Here's the drawing with two shaded views (mm, measured from the low corner). I have some questions. Coordinates: 2 decimals unless noted, no trailing zeros. Loops run counter-clockwise (first coordinate to the right, second up) from the corner with the lowest first, then second, coordinate; pieces in that order, holes last. Notation, with made-up numbers: (-36, 53) -> (1, 53) arc R16 cw to (1, 63) -> close; hole circle Ø3 at (89.5, 85.5). An arc over 180 degrees is marked (long way). Answer as a JSON object with one key per item and string values. Group by question number.
1) I want a section at A-A (y = 1.5). Write out the boundary of the cut face in (x, z).
2) I'm going to push a flat-ended pin straight in: pin 1 (1.5 mm diameter, centred on x = 48.5, y = 1.5, fed in from -Z). Where does the tip first touch, or does it pass through?
3) I need wall thicknesses on probe 1 along X at (y, z) = (1.05, 11); probe 2 along Z at (x, y) = (45, 0.45). Which ranges of each line are inside material? Lowest first, please. Write a range as [from, to].
4) I want a section at B-B (x = 84). Write out the boundary of the cut face in (y, z), then the cut area to 3 significant figures.
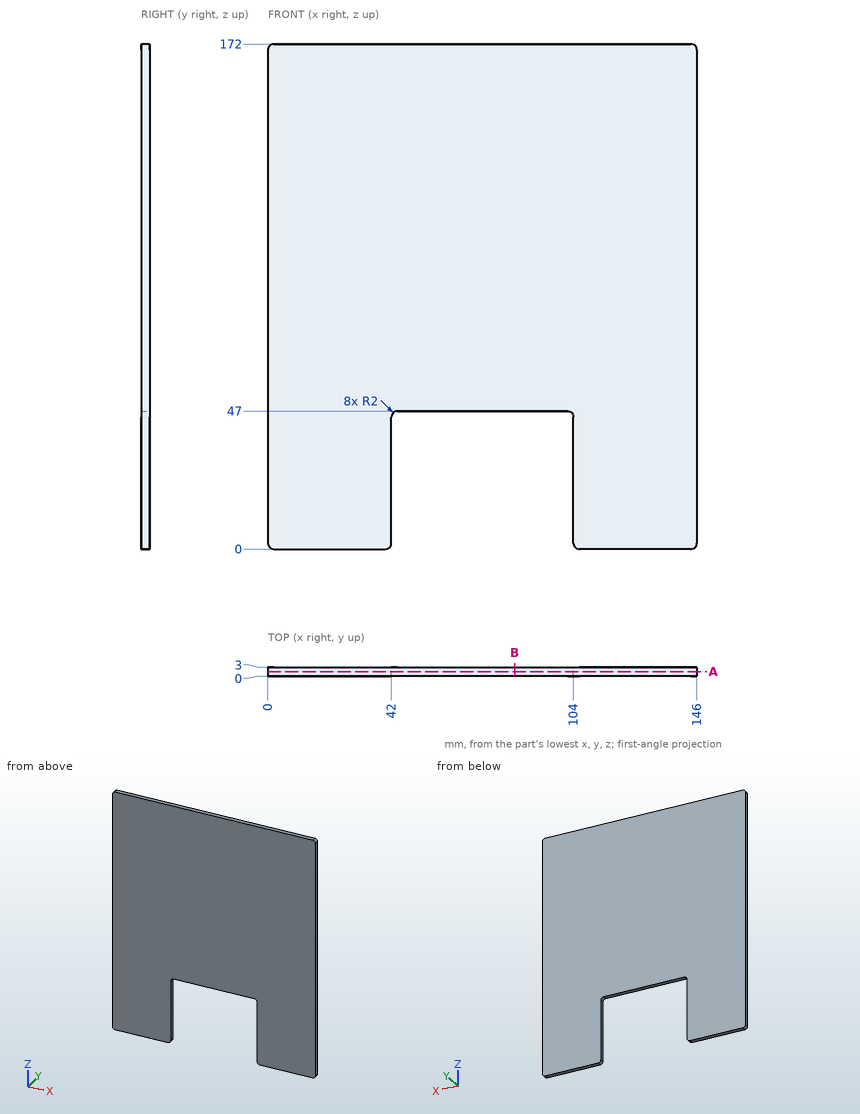
Determined:
{
 "1": {"outline": "(0, 2) arc R2 ccw to (2, 0) -> (40, 0) arc R2 ccw to (42, 2) -> (42, 45) arc R2 cw to (44, 47) -> (102, 47) arc R2 cw to (104, 45) -> (104, 2) arc R2 ccw to (106, 0) -> (144, 0) arc R2 ccw to (146, 2) -> (146, 170) arc R2 ccw to (144, 172) -> (2, 172) arc R2 ccw to (0, 170) -> close"},
 "2": {"pin 1": "z = 47"},
 "3": {"probe 1": "[0, 42], [104, 146]", "probe 2": "[47, 172]"},
 "4": {"outline": "(0, 47) -> (3, 47) -> (3, 172) -> (0, 172) -> close", "area": "375 mm^2"}
}
